The listing builds one solid part. Answer for the finished solid, in the listing's coordinates (mm). Face numbers are marked on the shaded views. A direction names the side the tool comes from. Coordinates: 2 decimals unless noted, no trailing zeros. Write each loop counter-clockwise with the first axis right and the second up, starting at its lowest first coordinate (ties: lowest second). Pieces come first, ordered by that corner, then holes. Notation, with made-up numbers: M 6.5,5.25 L 22.5,5.25 A18 cw 22.5,15.25 Z; hole C 0.25,36 d10. An arc over 180 degrees is marked long. Answer as a JSON object with one key per item and string values. Group by question number.
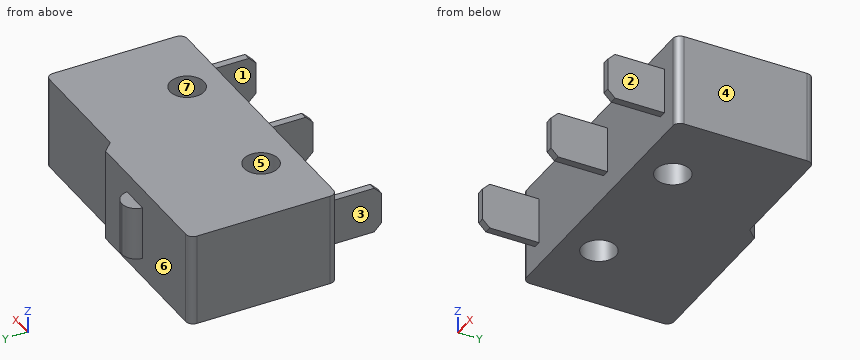
from build123d import *

# Parameters (mm, degrees)
SKETCH_1_W               = 19.8
SKETCH_1_H               = 10.2
EXTRUDE_1_DEPTH          = 6.4
CUT_EXTRUDE_1_DEPTH      = 13.844454056
CUT_EXTRUDE_1_DEPTH_BACK = 13.844454056
SKETCH_3_R               = 1.175
CUT_EXTRUDE_2_DEPTH      = 13.844454056
SKETCH_4_W               = 2
SKETCH_4_H               = 3.7
EXTRUDE_2_DEPTH          = 0.9
FILLET_2_R               = 0.5
FILLET_3_R               = 1
SKETCH_6_W               = 0.5
SKETCH_6_H               = 3.2
EXTRUDE_3_DEPTH          = 3.9
CHAMFER_1_SIZE           = 0.5


with BuildPart() as part:
    # 草图1 → 凸台-拉伸1 (new body)
    with BuildSketch(Plane.XY):
        Rectangle(SKETCH_1_W, SKETCH_1_H)
    extrude(amount=EXTRUDE_1_DEPTH)

    # 草图2 → 切除-拉伸1 (cut, two sides: drawn at the far end of the back side and taken through both)
    with BuildSketch(Plane.XY.offset(6.4).offset(-CUT_EXTRUDE_1_DEPTH_BACK)):
        Polygon((9.9, 5.1), (0.905266145, 5.1), (1.605266145, 4.4), (9.9, 4.4), align=None)
    extrude(amount=CUT_EXTRUDE_1_DEPTH + CUT_EXTRUDE_1_DEPTH_BACK, mode=Mode.SUBTRACT)

    # 草图3 → 切除-拉伸2 (cut, through all)
    with BuildSketch(Plane.XY.offset(6.4)):
        with Locations((-4.75, -2.6)):
            Circle(SKETCH_3_R)
        with Locations((4.75, -2.6)):
            Circle(SKETCH_3_R)
    extrude(amount=-CUT_EXTRUDE_2_DEPTH, mode=Mode.SUBTRACT)

    # 草图4 → 凸台-拉伸2 (add)
    with BuildSketch(Plane(origin=(0, 5.1, 0), x_dir=(1, 0, 0), z_dir=(0, 1, 0))):
        with Locations((-2.85, -3.2)):
            Rectangle(SKETCH_4_W, SKETCH_4_H)
    extrude(amount=EXTRUDE_2_DEPTH)

    # 圆角2
    fillet_2_edges = [part.edges().sort_by_distance(p)[0] for p in [
        (9.9, 4.4, 3.2),
        (-9.9, 5.1, 3.2),
        (9.9, -5.1, 3.2),
        (-9.9, -5.1, 3.2),
    ]]
    fillet(fillet_2_edges, radius=FILLET_2_R)

    # 圆角3
    # the kernel refuses this fillet: 1 mm, written as the material it takes off along each edge
    with BuildSketch(Plane(origin=(-1.85, 6, -1.137468593), x_dir=(0, -1, 0), z_dir=(0, 0, 1)), Plane(origin=(-3.85, 6, 7.537468593), x_dir=(0, -1, 0), z_dir=(0, 0, -1))) as fillet_3_piece_1:
        with BuildLine():
            CenterArc((1, -0.994987437), FILLET_3_R, 95.739170477, 84.260829523)
            Line((0, -0.994987437), (-0.02, -0.994987437))
            Line((-0.02, -0.994987437), (-0.02, 0))
            Line((-0.02, 0), (0, 0.02))
            ThreePointArc((0, 0.02), (0.45, 0.02), (0.898, 0.019899749))
            Line((0.898, 0.019899749), (0.9, 0))
        make_face()
    extrude(amount=8.674937186, mode=Mode.SUBTRACT)

    # 草图6 → 凸台-拉伸3 (add)
    with BuildSketch(Plane.XZ.offset(5.1)):
        with Locations((-8.05, 3.2)):
            Rectangle(SKETCH_6_W, SKETCH_6_H)
        with Locations((0.75, 3.2)):
            Rectangle(SKETCH_6_W, SKETCH_6_H)
        with Locations((8.05, 3.2)):
            Rectangle(SKETCH_6_W, SKETCH_6_H)
    extrude(amount=EXTRUDE_3_DEPTH)

    # 倒角1
    chamfer_1_edges = [part.edges().sort_by_distance(p)[0] for p in [
        (0.75, -9, 4.8),
        (0.75, -9, 1.6),
        (8.05, -9, 4.8),
        (8.05, -9, 1.6),
        (-8.05, -9, 4.8),
        (-8.05, -9, 1.6),
    ]]
    chamfer(chamfer_1_edges, length=CHAMFER_1_SIZE)


solid = part.part
Item 1: A cutting plane is placed at D-D, the plane y = -5.5. Write down the section's boundary in (x, z), and give its area (3 significant figures).
Item 2: A cutting plane is placed at A-A, the plane x = 4.75. Write down the section's boundary in (y, z) (3 decimals), and give its area (3 significant figures).
Item 3: Flat-ended cylindrical pins translate along their axes: pin 1 Ø3.5 at (y, z) = (-6.5, 3) entering from -X; pin 2 Ø2.5 at (y, z) = (-8, 2.5) entering from -X; pin 3 Ø1 at (y, z) = (-6.5, 3) entering from +X. Find the tip coordinate at first contact, or state that the pin passes through.
Item 4: Consider L1, parallel to X at y = -2.5, z = 4.25; L2, parallel to X at y = -6.75, z = 3.75; L3, parallel to Y at x = -4.75, z = 3.5 (3 decimals). Determine where each line is inside the solid, lowest interval first. Write a range as from..to.
Item 5: A cutting plane is placed at C-C, the plane z = 0.5. Write down the section's boundary in (x, y) (3 decimals), and give its area (3 significant figures).
Item 6: A tool of negligible diameter and unlimited length cuts with its end or side. For the marked faces 1, 2 and 3, from which of +Z, -Z, +X, -X, +Y, -Y can it reach the whole face along a straight path? Write none if from no direction.
Item 7: For a pull along Y with two mould halves and no side action, classify the marked faces 4, 5, 6 and 7 as +Y half, -Y half, draft (parallel to the pull), parting line (faces both ways), or undercut.
Item 8: A cutting plane is placed at B-B, the plane y = -2.6. Write down the section's boundary in (x, z) (3 decimals).
Answer:
{
 "1": {"outline": "M -8.3,1.6 L -7.8,1.6 L -7.8,4.8 L -8.3,4.8 Z; M 0.5,1.6 L 1,1.6 L 1,4.8 L 0.5,4.8 Z; M 7.8,1.6 L 8.3,1.6 L 8.3,4.8 L 7.8,4.8 Z", "area": "4.80 mm2"},
 "2": {"outline": "M -5.1,0 L -3.775,0 L -3.775,6.4 L -5.1,6.4 Z; M -1.425,0 L 4.4,0 L 4.4,6.4 L -1.425,6.4 Z", "area": "45.8 mm2"},
 "3": {"pin 1": "x = -9.88", "pin 2": "x = -8.3", "pin 3": "x = 8.3"},
 "4": {"L1": "-9.9..-5.92, -3.58..3.58, 5.92..9.9", "L2": "-8.3..-7.8, 0.5..1, 7.8..8.3", "L3": "-5.1..-3.775, -1.425..5.1"},
 "5": {"outline": "M -9.9,-4.6 A0.5 ccw -9.4,-5.1 L 9.4,-5.1 A0.5 ccw 9.9,-4.6 L 9.9,3.9 A0.5 ccw 9.4,4.4 L 1.605,4.4 L 0.905,5.1 L -9.4,5.1 A0.5 ccw -9.9,4.6 Z; hole C -4.75,-2.6 d2.35; hole C 4.75,-2.6 d2.35", "area": "187 mm2"},
 "6": {"face 1": "+Z, -Z, -Y", "face 2": "+Z, -Z, +X, -Y", "face 3": "+Z, -Z, -X, -Y"},
 "7": {"face 4": "draft", "face 5": "undercut", "face 6": "+Y half", "face 7": "undercut"},
 "8": {"outline": "M -9.9,0 L -5.925,0 L -5.925,6.4 L -9.9,6.4 Z; M -3.575,0 L 3.575,0 L 3.575,6.4 L -3.575,6.4 Z; M 5.925,0 L 9.9,0 L 9.9,6.4 L 5.925,6.4 Z"}
}
